Autodesk Inventor part; units mm, degrees
ref_plane "YZ Plane" through (0, 0, 0) normal (1, 0, 0) x (0, 1, 0)
ref_plane "XZ Plane" through (0, 0, 0) normal (0, 1, 0) x (-1, 0, 0)
ref_plane "XY Plane" through (0, 0, 0) normal (0, 0, 1) x (1, 0, 0)
sketch "Sketch1" plane through (0, 0, 0) normal (0, 0, 1) x (1, 0, 0)
  line L0 (252.3, 12.7) -> (0.0018, 12.7)
  line L1 (0.0018, 12.7) -> (0.0018, 28.399)
  line L2 (0.0018, 28.399) -> (103.5611, 28.399)
  line L3 (252.3, 28.399) -> (252.3, 12.7)
  line L4 (252.3, 190.5) -> (103.5611, 28.399)
  line L5 (252.3, 28.399) -> (252.3, 190.5)
  point P0 (0, 0)
  point P1 (0, 12.7)
  dimension "d2" = 220
extrude "Extrusion1" add sketch "Sketch1" against normal blind 12.7
Part model, mm, in its own coordinate system. A direction names the side the tool comes from. Give positions to 0.01 mm unless a question says otherwise; leave off trailing zeros. Order: outer loops, then holes, each group sorted by start corner. A loop starts at its lowest first (then second) coordinate and runs counter-clockwise, first axis right, second up. Notation, with made-up numbers: (-4, 5.25) -> (25, 5.25) arc R7 ccw to (25, 18.25) -> close; hole circle Ø6 at (22.5, -12). An arc over 180 degrees is marked (long way). Use one line per item in the form item = value.
(1) Flat gauge pins, fed straight in: P1, Ø3, axis at y = 61, z = -1.5, coming from the -X side; P2, Ø5, axis at y = 106, z = -6, coming from the -X side; P3, Ø2, axis at y = 137.5, z = -8, coming from the -X side. Where does each tip first touch, or does it go through?
Solution:
P1 = 132.1
P2 = 172.47
P3 = 202.75
(2) Drill centre lines: line 1 (Y direction, x = 99, z = -10.75); line 2 (X direction, y = 40.5, z = -10.5); line 3 (X direction, y = 94, z = -9). Where is each one in solid material? Low to high. Write a range as from..to.
Solution:
line_1 = 12.7..28.4
line_2 = 114.66..252.3
line_3 = 163.75..252.3
(3) Tool access for faces 1 (the face through (51, 28.399, -6)), 2 (the face through (128, 12.7, -6)): list every direction of +Z, -Z, +X, -X, +Y, -Y with a clear straight run to the whole face (end or side of a thin tool).
Solution:
face_1 = +Z, -Z, -X, +Y
face_2 = +Z, -Z, +X, -X, -Y
(4) Saw through at C-C (x = 24). Write the cut outline in (y, z), then the cut area to 3 significant figures.
Solution:
outline = (12.7, -12.7) -> (28.4, -12.7) -> (28.4, 0) -> (12.7, 0) -> close
area = 199 mm²
(5) Saw through at A-A (z = -8). Write the cut outline in (x, y), then the cut area to 3 significant figures.
Solution:
outline = (0, 12.7) -> (252.3, 12.7) -> (252.3, 190.5) -> (103.56, 28.4) -> (0, 28.4) -> close
area = 16,000 mm²
(6) Saw through at B-B (y = 129). Write the cut outline in (x, z).
Solution:
outline = (195.87, -12.7) -> (252.3, -12.7) -> (252.3, 0) -> (195.87, 0) -> close
